Design review of the part built by this model. Coordinates are the model's own, in mm. A direction names the side the tool comes from. Coordinates: 2 decimals unless noted, no trailing zeros. Loops run counter-clockwise (first coordinate to the right, second up) from the corner with the lowest first, then second, coordinate; pieces in that order, holes last.
from build123d import *

# Parameters (mm, degrees)
BOSS_EXTRUDE1_DEPTH     = 4
CUT_EXTRUDE1_DEPTH      = 16.297058541
CUT_EXTRUDE1_DEPTH_BACK = 16.297058541
SKETCH2_W               = 2.2
SKETCH2_H               = 3
SKETCH3_W               = 1
SKETCH3_H               = 3
CUT_EXTRUDE2_DEPTH      = 16.297058541


with BuildPart() as part:
    # Sketch1 → Boss-Extrude1 (new, symmetric)
    with BuildSketch(Plane(origin=(0, 0, 0), x_dir=(1, 0, 0), z_dir=(0, 1, 0))):
        Polygon((-7, 13), (-7, 6), (-4.25, 0), (4.25, 0), (7, 6), (7, 13), (2.95, 13), (2.95, 5), (-2.95, 5), (-2.95, 13), align=None)
    extrude(amount=BOSS_EXTRUDE1_DEPTH, both=True)

    # Sketch2 → Cut-Extrude1 (cut, two sides: drawn at the far end of the back side and taken through both)
    with BuildSketch(Plane(origin=(0, 0, 0), x_dir=(0, 0, -1), z_dir=(1, 0, 0)).offset(-CUT_EXTRUDE1_DEPTH_BACK)):
        with Locations((1.1, 0)):
            Rectangle(SKETCH2_W, SKETCH2_H)
    extrude(amount=CUT_EXTRUDE1_DEPTH + CUT_EXTRUDE1_DEPTH_BACK, mode=Mode.SUBTRACT)

    # Sketch3 → Cut-Extrude2 (cut, through all)
    with BuildSketch(Plane.XY):
        with Locations((-6.5, 0)):
            Rectangle(SKETCH3_W, SKETCH3_H)
        with Locations((6.5, 0)):
            Rectangle(SKETCH3_W, SKETCH3_H)
    extrude(amount=-CUT_EXTRUDE2_DEPTH, mode=Mode.SUBTRACT)


solid = part.part
Q1. The part is to be moulded in two halves that separate along Y. For faces 5 (the flat face through (6, 0, -8)), 6 (the flat face through (-7, 3, -10)), say which applies: pulls with the +Y half, pulls with the -Y half, needs draft (parallel to the pull), parting line crosses it, or undercut.
Q2. For line 1 (X direction, y = 1.25, z = -8.25); line 2 (X direction, y = -3.5, z = -9.75); line 3 (Z direction, x = 2.75, y = -1.75), list the stretches that pass through material, from the lowest coordinate up.
Q3. Take a section at A-A, the plane z = -8. Write out the cut boundary in (x, y).
Q4. Take a section at B-B, the plane x = -2.5. Write out the cut boundary in (y, z).
Q5. Take a section at C-C, the plane y = -2.5. Write out the cut boundary in (x, z).
Q6. Clearance check with flat-ended pins moving along their axes: pin 1 Ø4 at (y, z) = (3, -2.5) entering from +X; pin 2 Ø1.5 at (x, y) = (1.5, 0.5) entering from +Z; pin 3 Ø1 at (x, y) = (2, -3) entering from -Z. State where each tip first meets the part, or that it passes through.
Q7. Take a section at D-D, the plane z = -4. Write out the cut boundary in (x, y).
Q8. Machinability: for faces 1 (the flat face through (0, -1.5, -1)), 2 (the flat face through (6.5, -1.5, -9.4)), 3 (the flat face through (2.95, 0, -9)), 4 (the flat face through (-6.5, -1.5, -9.4)), which of the approach directions +Z, -Z, +X, -X, +Y, -Y give a long, thin tool a straight path to every point of the face, cutting with its end or side? Answer none if there is none.
Entries:
1. face 5: undercut
1. face 6: needs draft
2. line 1: x = -6 to -2.95, 2.95 to 6
2. line 2: x = -7 to -2.95, 2.95 to 7
2. line 3: z = -5 to 0
3. outline: (-7, -4) - (-2.95, -4) - (-2.95, 4) - (-7, 4) - (-7, 1.5) - (-6, 1.5) - (-6, -1.5) - (-7, -1.5) - close; (2.95, -4) - (7, -4) - (7, -1.5) - (6, -1.5) - (6, 1.5) - (7, 1.5) - (7, 4) - (2.95, 4) - close
4. outline: (-4, -5) - (4, -5) - (4, 0) - (1.5, 0) - (1.5, -2.2) - (-1.5, -2.2) - (-1.5, 0) - (-4, 0) - close
5. outline: (-7, -13) - (-2.95, -13) - (-2.95, -5) - (2.95, -5) - (2.95, -13) - (7, -13) - (7, -6) - (4.25, 0) - (-4.25, 0) - (-7, -6) - close
6. pin 1: stops at x = 6.31
6. pin 2: stops at z = -2.2
6. pin 3: stops at z = -5
7. outline: (-6.08, -4) - (6.08, -4) - (6.08, -1.5) - (6, -1.5) - (6, 1.5) - (6.08, 1.5) - (6.08, 4) - (-6.08, 4) - (-6.08, 1.5) - (-6, 1.5) - (-6, -1.5) - (-6.08, -1.5) - close
8. face 1: +Z, +X, -X
8. face 2: +Z, -Z, +X
8. face 3: -Z, +Y, -Y
8. face 4: +Z, -Z, -X
